The listing builds one solid part. Answer for the finished solid, in the listing's coordinates (mm). Coordinates: 2 decimals unless noted, no trailing zeros. Write each loop counter-clockwise with the first axis right and the second up, starting at its lowest first coordinate (ties: lowest second). Pieces come first, ordered by that corner, then holes. Notation, with made-up numbers: M 10,24.5 L 67,24.5 A12 cw 67,42.5 Z; hole C -1,20.25 d5. An arc over 180 degrees is marked long. Put each result on its own line as item: value. Start each with the question number.
```python
from build123d import *

# Parameters (mm, degrees)
SKETCH1_W                = 185.42
SKETCH1_H                = 241.3
BOSS_EXTRUDE1_DEPTH      = 3.175
CUT_EXTRUDE1_OUTLINE_R   = 4.49453
CUT_EXTRUDE1_OUTLINE_R_2 = 1.0922
CUT_EXTRUDE1_DEPTH       = 3.175
CUT_EXTRUDE2_DEPTH       = 305.329339737
SKETCH8_R                = 1
SKETCH8_W                = 3.302
SKETCH8_H                = 7.874
CUT_EXTRUDE4_DEPTH       = 305.329339737
SKETCH9_W                = 76.2
SKETCH9_H                = 3.175
CUT_EXTRUDE5_DEPTH       = 305.329339737
SKETCH10_W               = 3.175
SKETCH10_H               = 76.2
BOSS_EXTRUDE4_DEPTH      = 3.175


# Read off the part's stored shape, not the designer's step: Cut-Extrude1
with BuildPart() as part:
    # Sketch1 → Boss-Extrude1 (new body)
    with BuildSketch(Plane(origin=(0, 0, 0), x_dir=(1, 0, 0), z_dir=(0, 1, 0))):
        with Locations((92.71, 120.65)):
            Rectangle(SKETCH1_W, SKETCH1_H)
    extrude(amount=BOSS_EXTRUDE1_DEPTH)

    # Cut-Extrude1 outline → Cut-Extrude1 (cut)
    with BuildSketch(Plane(origin=(0, 0, 0), x_dir=(1, 0, 0), z_dir=(0, 1, 0))):
        with Locations((145.415, 120.65)):
            Circle(CUT_EXTRUDE1_OUTLINE_R)
        with Locations((153.338312588, 128.573312588)):
            Circle(CUT_EXTRUDE1_OUTLINE_R_2)
        with Locations((137.491687412, 128.573312588)):
            Circle(CUT_EXTRUDE1_OUTLINE_R_2)
        with Locations((137.491687412, 112.726687412)):
            Circle(CUT_EXTRUDE1_OUTLINE_R_2)
        with Locations((153.338312588, 112.726687412)):
            Circle(CUT_EXTRUDE1_OUTLINE_R_2)
    extrude(amount=CUT_EXTRUDE1_DEPTH, mode=Mode.SUBTRACT)

    # Sketch6 → Cut-Extrude2 (cut, through all)
    with BuildSketch(Plane(origin=(0, 3.175, 0), x_dir=(1, 0, 0), z_dir=(0, 1, 0))):
        with BuildLine():
            Line((150.615, 64.796000096), (150.615, 74.496000096))
            ThreePointArc((150.615, 74.496000096), (152.115, 75.996000096), (153.615, 74.496000096))
            Line((153.615, 74.496000096), (153.615, 64.796000096))
            ThreePointArc((153.615, 64.796000096), (152.115, 63.296000096), (150.615, 64.796000096))
        make_face()
        with BuildLine():
            Line((159.515, 64.796000096), (159.515, 74.496000096))
            ThreePointArc((159.515, 74.496000096), (161.015, 75.996000096), (162.515, 74.496000096))
            Line((162.515, 74.496000096), (162.515, 64.796000096))
            ThreePointArc((162.515, 64.796000096), (161.015, 63.296000096), (159.515, 64.796000096))
        make_face()
    extrude(amount=-CUT_EXTRUDE2_DEPTH, mode=Mode.SUBTRACT)

    # Sketch8 → Cut-Extrude4 (cut, through all)
    with BuildSketch(Plane.XZ):
        with Locations(Location((175.895, -193.548, 0), (0, 0, 270))):
            Circle(SKETCH8_R)
        with Locations(Location((175.895, -210.058, 0), (0, 0, 90))):
            Circle(SKETCH8_R)
        with Locations((175.895, -201.803)):
            Rectangle(SKETCH8_W, SKETCH8_H)
    extrude(amount=-CUT_EXTRUDE4_DEPTH, mode=Mode.SUBTRACT)

    # Sketch9 → Cut-Extrude5 (cut, through all)
    with BuildSketch(Plane(origin=(0, 3.175, 0), x_dir=(1, 0, 0), z_dir=(0, 1, 0))):
        with Locations((92.71, 239.7125)):
            Rectangle(SKETCH9_W, SKETCH9_H)
        with Locations((92.71, 1.5875)):
            Rectangle(SKETCH9_W, SKETCH9_H)
    extrude(amount=-CUT_EXTRUDE5_DEPTH, mode=Mode.SUBTRACT)

    # Sketch10 → Boss-Extrude4 (add)
    with BuildSketch(Plane(origin=(0, 3.175, 0), x_dir=(1, 0, 0), z_dir=(0, 1, 0))):
        with Locations((-1.5875, 120.65)):
            Rectangle(SKETCH10_W, SKETCH10_H)
    extrude(amount=-BOSS_EXTRUDE4_DEPTH)


solid = part.part
```
1) Straight lines are drawn through the part: probe 1 along X at (y, z) = (2.8, -70) (3 decimals); probe 2 along X at (y, z) = (1.4, -120.65) (3 decimals); probe 3 along X at (y, z) = (1.85, -25.5). For each, find the intervals that lie inside material, in ascending order.
2) Determine the mould class of faces 1 (the face through (90, 0, -122)), 2 (the face through (140.925, 1.565, -120.848)) for opening direction X: +X half, -X half, draft (parallel to the pull), parting line (faces both ways), or undercut.
3) A cutting plane is placed at A-A on z = -120.65. Write down the section's boundary in (x, y) (3 decimals).
4) A cutting plane is placed at B-B on x = 121. Write down the section's boundary in (y, z) (3 decimals), then the cut area to 3 significant figures.
5) A cutting plane is placed at C-C on z = -219. Write down the section's boundary in (x, y) (3 decimals), then the cut area to 3 significant figures.
6) Given pin 1 Ø3 at (x, z) = (134.5, -122) entering from -Y; pin 2 Ø1.6 at (x, y) = (-2.5, 1.5) entering from +Z; pin 3 Ø1.3 at (x, z) = (137.49, -128.57) entering from -Y, each flat-ended and moving along its own axis, determine where each tip first touches the part or whether it passes through.
7) A cutting plane is placed at D-D on y = 1.6. State how many separate pieces and enclosed holes the cut face has, then the cut area to 3 significant figures.
Answers follow:
1. probe 1: x = 0 to 150.615, 153.615 to 159.515, 162.515 to 185.42
1. probe 2: x = -3.175 to 140.92, 149.91 to 185.42
1. probe 3: x = 0 to 185.42
2. face 1: draft
2. face 2: undercut
3. outline: M -3.175,0 L 140.92,0 L 140.92,3.175 L -3.175,3.175 Z; M 149.91,0 L 185.42,0 L 185.42,3.175 L 149.91,3.175 Z
4. outline: M 0,-238.125 L 3.175,-238.125 L 3.175,-3.175 L 0,-3.175 Z
4. area: 746 mm²
5. outline: M 0,0 L 185.42,0 L 185.42,3.175 L 0,3.175 Z
5. area: 589 mm²
6. pin 1: stops at y = 0
6. pin 2: stops at z = -82.55
6. pin 3: passes through
7. separate pieces: 1
7. enclosed holes: 10
7. area: 44,300 mm²
